The listing builds one solid part. Answer for the finished solid, in the listing's coordinates (mm). A direction names the side the tool comes from. Round coordinates to 2 decimals unless told otherwise and drop trailing zeros. Loops run counter-clockwise (first coordinate to the right, second up) from the corner with the lowest first, then second, coordinate; pieces in that order, holes last. Notation, with made-up numbers: (-26.5, 59.25) -> (30.5, 59.25) arc R12 cw to (30.5, 82.25) -> close; hole circle Ø7 at (59, 56). An arc over 180 degrees is marked (long way). Use a Markdown table: item, result. Add a question column.
Q1. Section B-B on y = -19 is taken. Give the vertices of the cut face in (x, z), then the cut area to 3 significant figures.
Q2. Given pin 1 Ø3 at (x, y) = (3.5, -12.5) entering from +Z; pin 2 Ø1 at (x, z) = (4, 11.5) entering from -Y, each flat-ended and moving along its own axis, determine where each tip first touches the part or whether it passes through.
Q3. Section D-D on z = 20 is taken. Give the number of separate pieces and of enclosed holes in the cut face, then the cut area to 3 significant figures.
Q4. Section C-C on x = 3.5 is taken. Give the vertices of the cut face in (y, z), then the cut area to 3 significant figures.
Q5. Consider line 1 (Y direction, x = 10.25, z = 8.5); line 2 (X direction, y = -11.5, z = 14.25); line 3 (Z direction, x = 2.25, y = 19). Determine where each line is inside the solid, lowest interval first.
Q6. Which of the six approach directions +Z, -Z, +X, -X, +Y, -Y give full straight-line access (tool end or side, diameter ignored) to faces 3 (the flat face through (0, 17, 1)), 4 (the cylindrical face through (-11.012, -25.493, 0.892)), 5 (the flat face through (11.5, -26, 20))?
Q7. For a pull along X with two mould halves and no side action, classify faces 1 (the flat face through (0, 0, 0)), 2 (the flat face through (-11.5, -8, 11)) as released by +X, released by -X, zero draft, split by the parting line, or undercut.
Q8. Section A-A on z = 4 is taken. Give the vertices of the cut face in (x, y), then the cut area to 3 significant figures.
from build123d import *

# Parameters (mm, degrees)
SKETCH_1_W          = 25
SKETCH_1_H          = 50
EXTRUDE_1_DEPTH     = 21
SKETCH_2_W          = 23
SKETCH_2_H          = 15
SKETCH_2_H_2        = 30
CUT_EXTRUDE_1_DEPTH = 20
SKETCH_3_R          = 0.5
EXTRUDE_2_DEPTH     = 1
FILLET_1_R          = 0.5


with BuildPart() as part:
    # 草圖1 → 填料-伸長1 (new body)
    with BuildSketch(Plane.XY):
        Rectangle(SKETCH_1_W, SKETCH_1_H)
    extrude(amount=EXTRUDE_1_DEPTH)

    # 草圖2 → 除料-伸長1 (cut)
    with BuildSketch(Plane.XY.offset(21)):
        with Locations((0, 16.5)):
            Rectangle(SKETCH_2_W, SKETCH_2_H)
        with Locations((0, -8)):
            Rectangle(SKETCH_2_W, SKETCH_2_H_2)
    extrude(amount=-CUT_EXTRUDE_1_DEPTH, mode=Mode.SUBTRACT)

    # 草圖3 → 填料-伸長2 (add)
    with BuildSketch(Plane.XZ.offset(25)):
        with Locations(Location((-11.5, 20, 0), (0, 0, 90))):
            Circle(SKETCH_3_R)
        with Locations(Location((11.5, 20, 0), (0, 0, 90))):
            Circle(SKETCH_3_R)
        with Locations(Location((11.5, 1, 0), (0, 0, 90))):
            Circle(SKETCH_3_R)
        with Locations(Location((-11.5, 1, 0), (0, 0, 90))):
            Circle(SKETCH_3_R)
    extrude(amount=EXTRUDE_2_DEPTH)

    # 圓角1
    fillet_1_edges = [part.edges().sort_by_distance(p)[0] for p in [
        (0, -25, 0),
        (-12.5, 0, 0),
        (0, 25, 0),
        (12.5, 0, 0),
        (12.5, -25, 10.5),
        (-12.5, -25, 10.5),
        (-12.5, 25, 10.5),
        (12.5, 25, 10.5),
    ]]
    fillet(fillet_1_edges, radius=FILLET_1_R - 0.0001)  # a hair under: the kernel refuses the full size


solid = part.part
Checked values:
| question | item | result |
|---|---|---|
| 1 | outline | (-12.5, 0.5) arc R0.5 ccw to (-12, 0) -> (12, 0) arc R0.5 ccw to (12.5, 0.5) -> (12.5, 21) -> (11.5, 21) -> (11.5, 1) -> (-11.5, 1) -> (-11.5, 21) -> (-12.5, 21) -> close |
| 1 | area | 64.9 mm2 |
| 2 | pin 1 | stops at z = 1 |
| 2 | pin 2 | stops at y = -25 |
| 3 | separate pieces | 1 |
| 3 | enclosed holes | 2 |
| 3 | area | 217 mm2 |
| 4 | outline | (-25, 0.5) arc R0.5 ccw to (-24.5, 0) -> (24.5, 0) arc R0.5 ccw to (25, 0.5) -> (25, 21) -> (24, 21) -> (24, 1) -> (9, 1) -> (9, 21) -> (7, 21) -> (7, 1) -> (-23, 1) -> (-23, 21) -> (-25, 21) -> close |
| 4 | area | 150 mm2 |
| 5 | line 1 | y = -25 to -23, 7 to 9, 24 to 25 |
| 5 | line 2 | x = -12.5 to -11.5, 11.5 to 12.5 |
| 5 | line 3 | z = 0 to 1 |
| 6 | face 3 | +Z |
| 6 | face 4 | -Y |
| 6 | face 5 | +Z, -Z, +X, -X, -Y |
| 7 | face 1 | zero draft |
| 7 | face 2 | undercut |
| 8 | outline | (-12.5, -24.5) arc R0.5 ccw to (-12, -25) -> (12, -25) arc R0.5 ccw to (12.5, -24.5) -> (12.5, 24.5) arc R0.5 ccw to (12, 25) -> (-12, 25) arc R0.5 ccw to (-12.5, 24.5) -> close; hole (-11.5, -23) -> (11.5, -23) -> (11.5, 7) -> (-11.5, 7) -> close; hole (-11.5, 9) -> (11.5, 9) -> (11.5, 24) -> (-11.5, 24) -> close |
| 8 | area | 215 mm2 |
